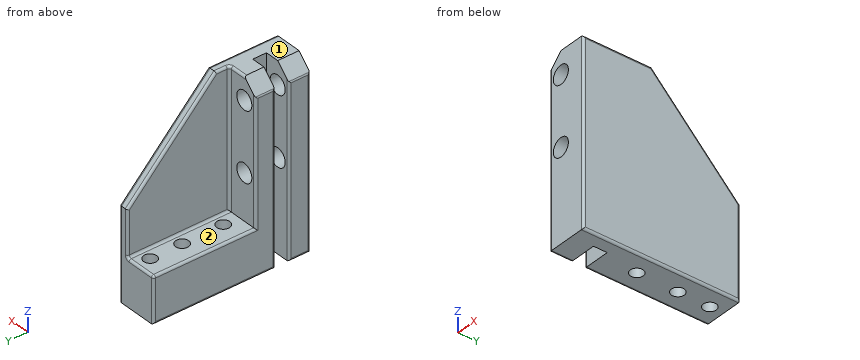
from build123d import *

# Parameters (mm, degrees)
SKETCH1_W           = 9
SKETCH1_H           = 34.4
SKETCH1_R           = 1.4224
BOSS_EXTRUDE1_DEPTH = 40
SKETCH1_3_R         = 1.4224
CUT_EXTRUDE1_DEPTH  = 10
SKETCH2_W           = 40
SKETCH2_H           = 3
CUT_EXTRUDE2_DEPTH  = 6
CUT_EXTRUDE3_DEPTH  = 9
CUT_EXTRUDE6_DEPTH  = 7
SKETCH6_R           = 2.0193
CUT_EXTRUDE5_DEPTH  = 20
FILLET2_R           = 0.5
CHAMFER4_SIZE       = 3
SKETCH7_W           = 74.310151154
SKETCH7_H           = 95.165931092
CUT_EXTRUDE7_DEPTH  = 9
FILLET3_R           = 0.5


with BuildPart() as part:
    # Sketch1 → Boss-Extrude1 (new body)
    with BuildSketch(Plane.XY):
        with Locations((4.5, 17.2)):
            Rectangle(SKETCH1_W, SKETCH1_H)
        with Locations((4.5, 15.4)):
            Circle(SKETCH1_R, mode=Mode.SUBTRACT)
        with Locations((4.5, 24.4)):
            Circle(SKETCH1_R, mode=Mode.SUBTRACT)
        with Locations((4.5, 24.4)):
            Circle(SKETCH1_R)
        with Locations((4.5, 15.4)):
            Circle(SKETCH1_R)
        with Locations((4.5, 31.4)):
            Circle(SKETCH1_R)
    extrude(amount=BOSS_EXTRUDE1_DEPTH)

    # Sketch1<3> → Cut-Extrude1 (cut)
    with BuildSketch(Plane.XY):
        with Locations((4.5, 24.4)):
            Circle(SKETCH1_3_R)
        with Locations((4.5, 31.4)):
            Circle(SKETCH1_3_R)
        with Locations((4.5, 15.4)):
            Circle(SKETCH1_3_R)
    extrude(amount=CUT_EXTRUDE1_DEPTH, mode=Mode.SUBTRACT)

    # Sketch2 → Cut-Extrude2 (cut)
    with BuildSketch(Plane(origin=(9, 0, 0), x_dir=(0, 0, -1), z_dir=(1, 0, 0))):
        with Locations((-20, 6.2)):
            Rectangle(SKETCH2_W, SKETCH2_H)
    extrude(amount=-CUT_EXTRUDE2_DEPTH, mode=Mode.SUBTRACT)

    # Sketch3 → Cut-Extrude3 (cut)
    with BuildSketch(Plane(origin=(9, 0, 0), x_dir=(0, 0, -1), z_dir=(1, 0, 0))):
        Polygon((-20, 34.4), (-40, 15), (-48.379363257, 51.913157268), align=None)
    extrude(amount=-CUT_EXTRUDE3_DEPTH, mode=Mode.SUBTRACT)

    # Sketch5 → Cut-Extrude6 (cut)
    with BuildSketch(Plane.ZY.offset(-9)):
        Polygon((20, 34.4), (10, 34.4), (10, 12), (40, 12), (40, 15), align=None)
    extrude(amount=CUT_EXTRUDE6_DEPTH, mode=Mode.SUBTRACT)

    # Sketch6 → Cut-Extrude5 (cut)
    with BuildSketch(Plane.XZ):
        with Locations((6, 35)):
            Circle(SKETCH6_R)
        with Locations((6, 20)):
            Circle(SKETCH6_R)
    extrude(amount=-CUT_EXTRUDE5_DEPTH, mode=Mode.SUBTRACT)

    # Fillet2
    fillet2_edges = [part.edges().sort_by_distance(p)[0] for p in [
        (0, 0, 20),
        (0, 7.5, 40),
        (0, 34.4, 10),
        (0, 24.7, 30),
        (0, 17.2, 0),
    ]]
    fillet(fillet2_edges, radius=FILLET2_R)

    # Chamfer4
    chamfer4_edges = [part.edges().sort_by_distance(p)[0] for p in [
        (9, 2.35, 40),
        (9, 9.85, 40),
    ]]
    chamfer(chamfer4_edges, length=CHAMFER4_SIZE)

    # Mirror1: part across plane


with BuildPart() as part_1:
    add(part.part)
    add(part.part.mirror(Plane(origin=(9, 0, 40), x_dir=(0, 0, 1), z_dir=(-1, 0, 0))))

    # Sketch7 → Cut-Extrude7 (cut)
    with BuildSketch(Plane.ZY):
        with Locations((29.906214843, 26.493385896)):
            Rectangle(SKETCH7_W, SKETCH7_H)
    extrude(amount=-CUT_EXTRUDE7_DEPTH, mode=Mode.SUBTRACT)

    # Fillet3
    fillet3_edges = [part_1.edges().sort_by_distance(p)[0] for p in [
        (16, 34.4, 15),
        (16, 13.5, 40),
        (14, 12, 40),
        (16, 24.7, 30),
        (16, 12, 25),
        (16, 23.2, 10),
        (9, 2.35, 37),
        (9, 9.85, 37),
        (12.5, 34.4, 10),
        (9, 2.35, 0),
        (9, 0, 18.5),
        (9, 4.7, 18.5),
        (9, 21.05, 0),
        (9, 7.7, 18.5),
        (9, 34.4, 5),
        (9, 23.2, 10),
        (9, 12, 23.5),
    ]]
    fillet(fillet3_edges, radius=FILLET3_R)


solid = part_1.part
Part model, mm, in its own coordinate system. Face numbers are marked on the shaded views. A direction names the side the tool comes from. Coordinates: 2 decimals unless noted, no trailing zeros. Loops run counter-clockwise (first coordinate to the right, second up) from the corner with the lowest first, then second, coordinate; pieces in that order, holes last. Notation, with made-up numbers: (89, 69) -> (137, 69) arc R22 cw to (137, 104) -> close; hole circle Ø6 at (2, 13.5). An arc over 180 degrees is marked (long way). Use a Markdown table: item, result. Add a question column.
Item 1: Band-saw the part on A-A on y = 13. Write the cut outline in (x, z).
Item 2: Which spindle directions (+Z, -Z, +X, -X, +Y, -Y) get a long thin tool onto all of the face, cutting with end or side? Do the marked faces 1 and 2. Say none if no direction does.
Item 3: Band-saw the part on B-B on z = 21. Give the number of separate pieces and of enclosed holes in the cut face, plus the area to 3 significant figures.
Item 4: Flat gauge pins, fed straight in: P1, Ø4.5, axis at x = 13.5, y = 31.4, coming from the +Z side; P2, Ø4.5, axis at x = 13.5, z = 24, coming from the +Y side; P3, Ø4.5, axis at x = 12, z = 20, coming from the +Y side. Where does each tip first touch, or does it go through?
Item 5: Probe probe 1 along Y at (x, z) = (13.5, 4.25); probe 2 along Y at (x, z) = (10.5, 10.5); probe 3 along Z at (x, y) = (11, 2). List the from-to ranges inside material, lowest first.
Geometry says:
| question | item | result |
|---|---|---|
| 1 | outline | (9, 0.5) arc R0.5 ccw to (9.5, 0) -> (17.5, 0) arc R0.5 ccw to (18, 0.5) -> (18, 39.5) arc R0.5 ccw to (17.5, 40) -> (16.5, 40) arc R0.5 ccw to (16, 39.5) -> (16, 10.5) arc R0.5 cw to (15.5, 10) -> (9.5, 10) arc R0.5 ccw to (9, 9.5) -> close |
| 2 | face 1 | +Z, +X, -X, +Y, -Y |
| 2 | face 2 | +Z, -X, +Y |
| 3 | separate pieces | 3 |
| 3 | enclosed holes | 0 |
| 3 | area | 101 mm² |
| 4 | P1 | z = 10.07 |
| 4 | P2 | y = 12.07 |
| 4 | P3 | y = 12 |
| 5 | probe 1 | 0 to 4.7, 7.7 to 13.98, 16.82 to 22.98, 25.82 to 29.98, 32.82 to 34.4 |
| 5 | probe 2 | 0 to 4.7, 7.7 to 12 |
| 5 | probe 3 | 0 to 18.25, 21.75 to 33.25, 36.75 to 39 |
